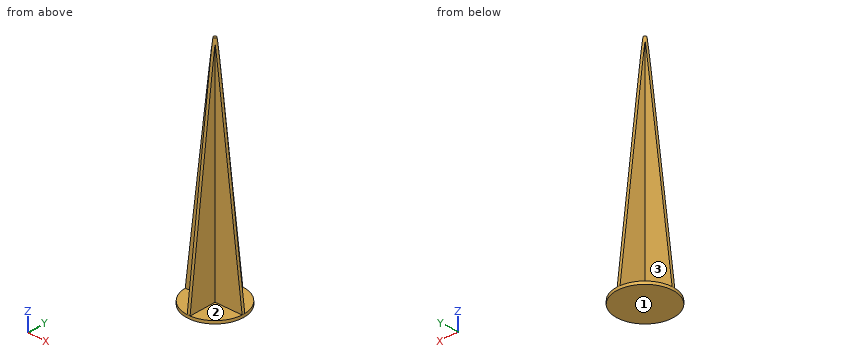
from build123d import *

# Parameters (mm, degrees)
CYLINDER_R     = 10
CYLINDER_DEPTH = 1
BOX001_W       = 20
BOX001_H       = 1
BOX001_DEPTH   = 80
BOX_W          = 20
BOX_H          = 1
BOX_DEPTH      = 80


with BuildPart() as cylinder:
    # Cylinder → Cylinder (new body)
    with BuildSketch(Plane.XY):
        Circle(CYLINDER_R)
    extrude(amount=CYLINDER_DEPTH)


with BuildPart() as cube001:
    # Box001 → Box001 (new body)
    with BuildSketch(Plane(origin=(0.5, -10, 0), x_dir=(0, 1, 0), z_dir=(0, 0, 1))):
        with Locations((10, 0.5)):
            Rectangle(BOX001_W, BOX001_H)
    extrude(amount=BOX001_DEPTH)


with BuildPart() as fusion:
    # Box → Box (new body)
    with BuildSketch(Plane(origin=(-10, -0.5, 0), x_dir=(1, 0, 0), z_dir=(0, 0, 1))):
        with Locations((10, 0.5)):
            Rectangle(BOX_W, BOX_H)
    extrude(amount=BOX_DEPTH)

    # Fusion: union Cube001
    add(cube001.part)


with BuildPart() as groundanchor:
    # Cone → Cone (revolve)
    with BuildSketch(Plane(origin=(0, 0, 1), x_dir=(1, 0, 0), z_dir=(0, -1, 0))):
        Polygon((0, 0), (10, 0), (0.4, 80), (0, 80), align=None)
    revolve(axis=Axis((0, 0, 1), (0, 0, 1)))

    # Common: intersect Fusion
    add(fusion.part, mode=Mode.INTERSECT)

    # Fusion001: union Cylinder
    add(cylinder.part)


solid = groundanchor.part
Could you check a few things on this model? Use its own coordinates, in mm. Face numbers are marked on the shaded views. A direction names the side the tool comes from. Give positions to 0.01 mm unless a question says otherwise; leave off trailing zeros. Loops run counter-clockwise (first coordinate to the right, second up) from the corner with the lowest first, then second, coordinate; pieces in that order, holes last. Notation, with made-up numbers: (77, 29) -> (135, 29) arc R22 ccw to (135, 39) -> close; hole circle Ø11 at (36.25, 58). An arc over 180 degrees is marked (long way). Return JSON: item names as keys, results as strings.
Item 1: If we section it at A-A on z = 75: List the corners of the cut face in (x, y) for me.
Geometry results:
{"outline": "(-1, -0.5) -> (-0.5, -0.5) -> (-0.5, -1) arc R1.12 ccw to (0.5, -1) -> (0.5, -0.5) -> (1, -0.5) arc R1.12 ccw to (1, 0.5) -> (0.5, 0.5) -> (0.5, 1) arc R1.12 ccw to (-0.5, 1) -> (-0.5, 0.5) -> (-1, 0.5) arc R1.12 ccw to start"}
Item 2: Which directions (+Z, -Z, +X, -X, +Y, -Y) give clear straight access to the entire face, cutting with the end or side of a thin tool? Please do the marked faces 1, 2 and 3.
Geometry results:
{"face 1": "-Z, +X, -X, +Y, -Y", "face 2": "+Z, +X, -Y", "face 3": "+Z, -X, +Y"}
Item 3: I'm going to push flat-ended pins straight in: pin 1 (7.5 mm diameter, centred on x = -6.5, y = 4.5, fed in from +Z); pin 2 (10.5 mm diameter, centred on x = -3.5, y = -3, fed in from +Z); pin 3 (10 mm diameter, centred on x = 3, z = 30, fed in from -Y); pin 4 (1 mm diameter, centred on x = -8, z = 34, fed in from +Y). Where does each tip first touch, or does it pass through?
Geometry results:
{"pin 1": "stops at z = 1", "pin 2": "stops at z = 80", "pin 3": "stops at y = -7.02", "pin 4": "passes through"}
Item 4: I need wall thicknesses on L1, parallel to Z at x = -4.25, y = 8.5; L2, parallel to X at y = 7.75, z = 11.5. Which ranges of each line are inside material? Lowest first, please. Write a range as from..to.
Geometry results:
{"L1": "z = 0..1", "L2": "x = -0.5..0.5"}
